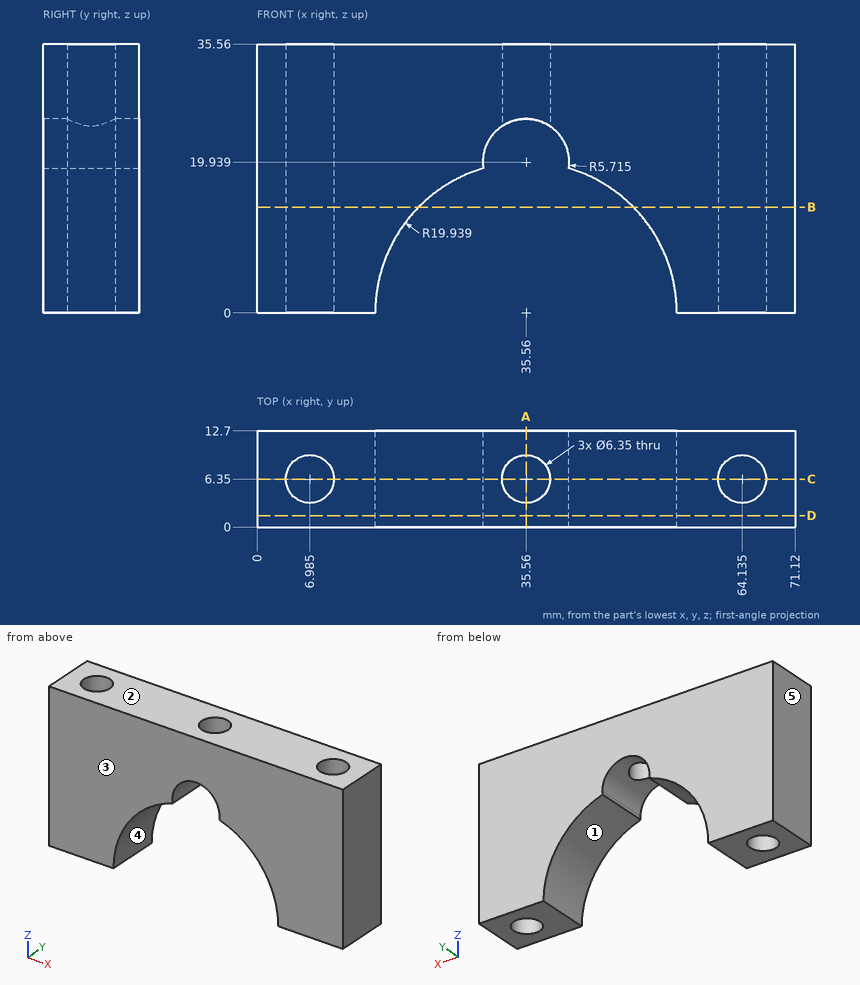
Study the drawing (mm; zero at the part's minimum x, y, z) and answer. A direction names the side the tool comes from. Round coordinates to 2 decimals unless told otherwise and drop trailing zeros. Loops run counter-clockwise (first coordinate to the right, second up) from the corner with the lowest first, then second, coordinate; pieces in that order, holes last. Notation, with made-up numbers: (-31.75, 57.25) -> (10.25, 57.25) arc R28 ccw to (10.25, 94.25) -> close; hole circle Ø1 at (-27.75, 52.5). An arc over 180 degrees is marked (long way). Write each question's results on one line, items separated by ' | '. Start each with the question number.
1. Section A-A (x = 35.56) is taken. Determine the outline of the cut face in (y, z) (3 decimals), plus the area to 3 significant figures.
2. Section D-D (y = 1.5) is taken. Determine the outline of the cut face in (x, z) (3 decimals), plus the area to 3 significant figures.
3. Find the intervals of material crossed by probe 1 along X at (y, z) = (7.5, 23); probe 2 along X at (y, z) = (4.75, 33); probe 3 along Y at (x, z) = (67, 12.5), in increasing order. Write a range as from..to.
4. Section C-C (y = 6.35) is taken. Determine the outline of the cut face in (x, z) (3 decimals).
5. A tool of negligible diameter and unlimited length cuts with its end or side. For the marked faces 1 and 2, from which of +Z, -Z, +X, -X, +Y, -Y can it reach the whole face along a straight path? Write none if from no direction.
6. Given pin 1 Ø7.5 at (x, y) = (64.135, 6.35) entering from -Z; pin 2 Ø4 at (x, y) = (35.56, 6.35) entering from -Z, each flat-ended and moving along its own axis, determine where each tip first touches the part or whether it passes through.
7. Section B-B (z = 14) is taken. Determine the outline of the cut face in (x, y) (3 decimals), plus the area to 3 significant figures.
8. For a pull along X with two mould halves and no side action, classify the marked faces 3, 4 and 5 as +X half, -X half, draft (parallel to the pull), parting line (faces both ways), or undercut.
Evaluation:
1) outline: (0, 25.654) -> (3.175, 25.654) -> (3.175, 35.56) -> (0, 35.56) -> close; (9.525, 25.654) -> (12.7, 25.654) -> (12.7, 35.56) -> (9.525, 35.56) -> close | area: 62.9 mm2
2) outline: (0, 0) -> (15.621, 0) arc R19.939 cw to (29.904, 19.12) arc R5.715 cw (long way) to (41.216, 19.12) arc R19.939 cw to (55.499, 0) -> (71.12, 0) -> (71.12, 35.56) -> (0, 35.56) -> close | area: 1,850 mm2
3) probe 1: x = 0..4.03, 9.94..30.73, 40.39..61.18, 67.09..71.12 | probe 2: x = 0..4.24, 9.73..32.82, 38.3..61.39, 66.88..71.12 | probe 3: y = 0..4.98, 7.72..12.7
4) outline: (0, 0) -> (3.81, 0) -> (3.81, 35.56) -> (0, 35.56) -> close; (10.16, 0) -> (15.621, 0) arc R19.939 cw to (29.904, 19.12) arc R5.715 cw to (32.385, 24.691) -> (32.385, 35.56) -> (10.16, 35.56) -> close; (38.735, 24.691) arc R5.715 cw to (41.216, 19.12) arc R19.939 cw to (55.499, 0) -> (60.96, 0) -> (60.96, 35.56) -> (38.735, 35.56) -> close; (67.31, 0) -> (71.12, 0) -> (71.12, 35.56) -> (67.31, 35.56) -> close
5) face 1: -Z, +Y, -Y | face 2: +Z, +X, -X, +Y, -Y
6) pin 1: stops at z = 0 | pin 2: passes through
7) outline: (0, 0) -> (21.363, 0) -> (21.363, 12.7) -> (0, 12.7) -> close; (49.757, 0) -> (71.12, 0) -> (71.12, 12.7) -> (49.757, 12.7) -> close; hole circle Ø6.35 at (6.985, 6.35); hole circle Ø6.35 at (64.135, 6.35) | area: 479 mm2
8) face 3: draft | face 4: undercut | face 5: -X half
